```python
from build123d import *

# Parameters (mm, degrees)
SKETCH1_W           = 190.5
SKETCH1_H           = 50.8
BOSS_EXTRUDE1_DEPTH = 6.35
SKETCH2_W           = 6.35
SKETCH2_H           = 12.7
CUT_EXTRUDE1_DEPTH  = 7.35
SKETCH3_W           = 6.35
SKETCH3_H           = 6.35
CUT_EXTRUDE2_DEPTH  = 7.35
SKETCH4_W           = 12.7
SKETCH4_H           = 6.35
CUT_EXTRUDE3_DEPTH  = 7.35
LPATTERN1_COUNT     = 7
LPATTERN1_PITCH     = 25.4


with BuildPart() as part:
    # Sketch1 → Boss-Extrude1 (new body)
    with BuildSketch(Plane.XY):
        Rectangle(SKETCH1_W, SKETCH1_H)
    extrude(amount=BOSS_EXTRUDE1_DEPTH)

    # Sketch2 → Cut-Extrude1 (cut, through all)
    with BuildSketch(Plane.XY.offset(6.35)):
        with Locations((-92.075, 0)):
            Rectangle(SKETCH2_W, SKETCH2_H)
    cut_extrude1 = extrude(amount=-CUT_EXTRUDE1_DEPTH, mode=Mode.SUBTRACT)

    # Sketch3 → Cut-Extrude2 (cut, through all)
    with BuildSketch(Plane.XY.offset(6.35)):
        with Locations((-92.075, -22.225)):
            Rectangle(SKETCH3_W, SKETCH3_H)
    cut_extrude2 = extrude(amount=-CUT_EXTRUDE2_DEPTH, mode=Mode.SUBTRACT)

    # Mirror1: Cut-Extrude2 across plane
    add(cut_extrude2.mirror(Plane(origin=(0, 0, 0), x_dir=(0, 0, 1), z_dir=(1, 0, 0))), mode=Mode.SUBTRACT)

    # Mirror2: Cut-Extrude1 across plane
    add(cut_extrude1.mirror(Plane(origin=(0, 0, 0), x_dir=(0, 0, 1), z_dir=(1, 0, 0))), mode=Mode.SUBTRACT)

    # Sketch4 → Cut-Extrude3 (cut, through all)
    with BuildSketch(Plane.XY.offset(6.35)):
        with Locations((-76.2, 22.225)):
            Rectangle(SKETCH4_W, SKETCH4_H)
    cut_extrude3 = extrude(amount=-CUT_EXTRUDE3_DEPTH, mode=Mode.SUBTRACT)

    # LPattern1: Cut-Extrude3 ×7
    with Locations(*[(i * LPATTERN1_PITCH, 0, 0) for i in range(1, LPATTERN1_COUNT)]):
        add(cut_extrude3, mode=Mode.SUBTRACT)


solid = part.part
```
Build history of the part. All positions in model axes, mm. A direction names the side the tool comes from. Coordinates: 2 decimals unless noted, no trailing zeros. Order: outer loops, then holes, each group sorted by start corner. A loop starts at its lowest first (then second) coordinate and runs counter-clockwise, first axis right, second up.
Item 1: Saw through at B-B on y = -22. List the corners of the cut face in (x, z), then the cut area to 3 significant figures.
Filled in:
outline: (-88.9, 0) - (88.9, 0) - (88.9, 6.35) - (-88.9, 6.35) - close
area: 1,130 mm2
Item 2: Tool access for faces 4 (the flat face through (92, -19.05, 3)), 5 (the flat face through (-92, -6.35, 3)), 6 (the flat face through (76, 19.05, 3)): list every direction of +Z, -Z, +X, -X, +Y, -Y with a clear straight run to the whole face (end or side of a thin tool).
Filled in:
face 4: +Z, -Z, +X, -Y
face 5: +Z, -Z, -X
face 6: +Z, -Z, +Y
Item 3: Mould opens along Y. For faces 1 (the flat face through (-92, -19.05, 3)), 2 (the flat face through (88.9, 0, 3)), 3 (the flat face through (-19.05, 22, 3)) say: released by +Y, released by -Y, zero draft, split by the parting line, or undercut.
Filled in:
face 1: released by -Y
face 2: undercut
face 3: zero draft
Item 4: Saw through at A-A on x = 73. List the corners of the cut face in (y, z), then the cut area to 3 significant figures.
Filled in:
outline: (-25.4, 0) - (19.05, 0) - (19.05, 6.35) - (-25.4, 6.35) - close
area: 282 mm2
Item 5: Drop flat-ended pins along their axis: pin 1 Ø1.9 at (x, z) = (-23.5, 3.5) entering from +Y; pin 2 Ø1.9 at (y, z) = (-23.5, 3) entering from +X; pin 3 Ø3 at (x, z) = (-93, 1.5) entering from -Y. Give the stop position or say it passes through.
Filled in:
pin 1: stops at y = 19.05
pin 2: stops at x = 88.9
pin 3: stops at y = -19.05
Item 6: Drill centre lines: L1, parallel to Y at x = -78.5, z = 3.25; L2, parallel to X at y = -2, z = 0.5. Where is each one in solid material? Low to high.
Filled in:
L1: y = -25.4 to 19.05
L2: x = -88.9 to 88.9
